Could you check a few things on this model? Use its own coordinates, in mm. Give positions to 0.01 mm unless a question says otherwise; leave off trailing zeros. One line per item, written item: value. Start each with the question number.
Q1. If I drill on line 1 (Y direction, x = 0.05, z = -5), over which ranges is the centre line in solid material (lowest first)? Write a range as from..to.
Q2. I'm going to push flat-ended pins straight in: P1, Ø0.6, axis at x = 0, z = 233.5, coming from the +Y side; P2, Ø0.5, axis at x = -0.5, z = 468.5, coming from the +Y side. Where does each tip first touch, or does it pass through?
Q3. I want a section at A-A (y = 34). Count the separate pieces of the cut face and the enclosed holes in it, then the cut area to 3 significant figures.
```python
from build123d import *

# Parameters (mm, degrees)
MIDDLE_DEPTH     = 0.8
LPATTERN3_COUNT  = 13
LPATTERN3_PITCH  = 33.333333
FIRST_DEPTH      = 0.8
FIRST_DEPTH_BACK = 0.8
LAST_DEPTH       = 0.8
LAST_DEPTH_BACK  = 0.8


with BuildPart() as part:
    # MiddlePart → Middle (new, symmetric)
    with BuildSketch(Plane(origin=(0, 0, 0), x_dir=(0, 0, -1), z_dir=(1, 0, 0))):
        Polygon((-33.333333, 23.59), (-33.333333, 0), (0, 0), (0, 23.59), (-0.64, 23.59), (-0.64, 47.5), (-32.693333, 47.5), (-32.693333, 23.59), align=None)
    extrude(amount=MIDDLE_DEPTH, both=True)

    # LPattern3: part ×13


with BuildPart() as part_1:
    add(part.part)
    with Locations(*[(0, 0, i * LPATTERN3_PITCH) for i in range(1, LPATTERN3_COUNT)]):
        add(part.part)

    # FirstPart → First (add, two sides: drawn at the far end of the back side and taken through both)
    with BuildSketch(Plane(origin=(0, 0, 0), x_dir=(0, 0, -1), z_dir=(1, 0, 0)).offset(-FIRST_DEPTH_BACK)):
        Polygon((0, 23.59), (0, 0), (54.8333355, 0), (54.8333355, 41.5), (3.64, 41.5), (3.64, 47.5), (0.64, 47.5), (0.64, 23.59), align=None)
    extrude(amount=FIRST_DEPTH + FIRST_DEPTH_BACK)

    # LastPart → Last (add, two sides: drawn at the far end of the back side and taken through both)
    with BuildSketch(Plane(origin=(0, 0, 0), x_dir=(0, 0, -1), z_dir=(1, 0, 0)).offset(-LAST_DEPTH_BACK)):
        Polygon((-436.973329, 47.5), (-433.973329, 47.5), (-433.973329, 23.59), (-433.333329, 23.59), (-433.333329, 0), (-488.1666645, 0), (-488.1666645, 41.5), (-436.973329, 41.5), align=None)
    extrude(amount=LAST_DEPTH + LAST_DEPTH_BACK)


solid = part_1.part
```
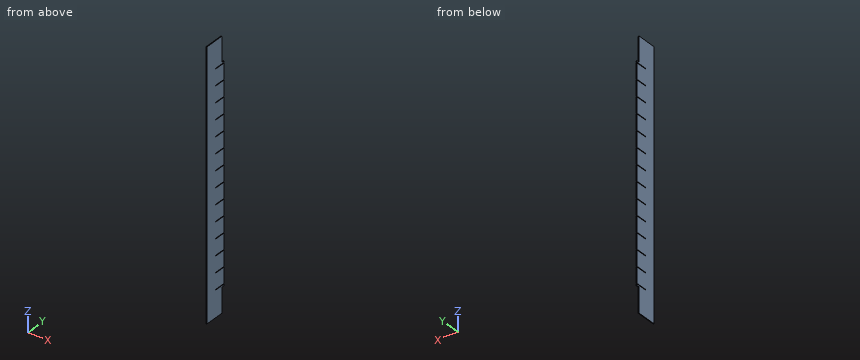
Worked answers:
1. line 1: y = 0..41.5
2. P1: stops at y = 23.59
2. P2: stops at y = 41.5
3. separate pieces: 15
3. enclosed holes: 0
3. area: 840 mm²
